Verification items for the finished model (mm, model axes). A direction names the side the tool comes from. Round coordinates to 2 decimals unless told otherwise and drop trailing zeros. Order: outer loops, then holes, each group sorted by start corner. A loop starts at its lowest first (then second) coordinate and runs counter-clockwise, first axis right, second up. Notation, with made-up numbers: M 42.25,44 L 67.25,44 A29 cw 67.25,64 Z; hole C 51,60 d1. An arc over 180 degrees is marked long. Return JSON: item names as keys, results as strings. Group by question number.
from build123d import *

# Parameters (mm, degrees)
BOSS_EXTRUDE1_DEPTH = 10
SKETCH1_3_R         = 7.5
BOSS_EXTRUDE2_DEPTH = 35
SKETCH3_W           = 111
SKETCH3_H           = 10
BOSS_EXTRUDE3_DEPTH = 300
SKETCH4_R           = 5
BOSS_EXTRUDE4_DEPTH = 15


with BuildPart() as part:
    # Sketch1 → Boss-Extrude1 (new body)
    with BuildSketch(Plane.XY):
        Polygon((30, 0), (30, 50), (-30, 50), (-30, 0), (-10.143306561, -30), (10.143306561, -30), align=None)
    boss_extrude1 = extrude(amount=BOSS_EXTRUDE1_DEPTH)

    # Sketch1_3 → Boss-Extrude2 (add)
    with BuildSketch(Plane.XY):
        Circle(SKETCH1_3_R)
    boss_extrude2 = extrude(amount=-BOSS_EXTRUDE2_DEPTH)

    # Sketch3 → Boss-Extrude3 (add)
    with BuildSketch(Plane.XY.offset(10)):
        with Locations((0, 55)):
            Rectangle(SKETCH3_W, SKETCH3_H)
    boss_extrude3 = extrude(amount=-BOSS_EXTRUDE3_DEPTH)

    # Mirror1: Boss-Extrude1, Boss-Extrude2, Boss-Extrude3 across plane
    add(boss_extrude1.mirror(Plane(origin=(0, 0, -290), x_dir=(1, 0, 0), z_dir=(0, 0, -1))))
    add(boss_extrude2.mirror(Plane(origin=(0, 0, -290), x_dir=(1, 0, 0), z_dir=(0, 0, -1))))
    add(boss_extrude3.mirror(Plane(origin=(0, 0, -290), x_dir=(1, 0, 0), z_dir=(0, 0, -1))))

    # Sketch4 → Boss-Extrude4 (add)
    with BuildSketch(Plane(origin=(0, 60, 0), x_dir=(1, 0, 0), z_dir=(0, 1, 0))):
        with Locations(Location((-45.5, -2.5, 0), (0, 0, 180))):
            Circle(SKETCH4_R)
        with Locations(Location((45.5, -2.5, 0), (0, 0, 180))):
            Circle(SKETCH4_R)
        with Locations(Location((-45.5, 552.5, 0), (0, 0, 180))):
            Circle(SKETCH4_R)
        with Locations(Location((45.5, 552.5, 0), (0, 0, 180))):
            Circle(SKETCH4_R)
    extrude(amount=BOSS_EXTRUDE4_DEPTH)


solid = part.part
1. Access from +Z, -Z, +X, -X, +Y, -Y to the whole of each face (thin tool, end or side, straight path). Record for faces 4 (the face through (30, 25, 5)), 5 (the face through (46.151, 67.395, -547.543)), 6 (the face through (-30, 25, 5)), 7 (the face through (-45, 75, -552)), 8 (the face through (55.5, 55, -294)).
2. Go/stop test with flat-tipped pins: pin 1 (3 mm diameter, centred on y = 18, z = 5.5, fed in from -X); pin 2 (6 mm diameter, centred on x = 8, z = -401, fed in from -Y); pin 3 (5 mm diameter, centred on y = 18, z = 5.5, fed in from +X). Record where each tip stops, or that it passes through.
3. Cross-section at A-A (z = -552.5). Enter the section's corners in (x, y), plus the area to 3 significant figures.
4. Draft check along Z on faces 1 (the face through (-1, 26, 10)), 2 (the face through (-30, 25, -585)), 3 (the face through (-7.493, 0.33, -562.745)). Enter one of: +Z half, -Z half, draft (parallel to the pull), parting line (faces both ways), or undercut.
5. Cross-section at D-D (y = 67). Enter the section's corners in (x, z).
6. Thickness scan on line 1 along Z through (x, y) = (13, -2.5); line 2 along Z through (x, y) = (-1, -4); line 3 along Y through (x, z) = (40.5, -496). Record the ranges inside material, lowest first. Write a range as from..to.
7. Cross-section at C-C (x = 45.5). Enter the section's corners in (y, z), plus the area to 3 significant figures.
8. Cross-section at B-B (y = 16). Enter the section's corners in (x, z).
Computed:
{
 "1": {"face 4": "+Z, -Z, +X, -Y", "face 5": "+Y", "face 6": "+Z, -Z, -X, -Y", "face 7": "+Z, -Z, +X, -X, +Y", "face 8": "+Z, -Z, +X, +Y, -Y"},
 "2": {"pin 1": "stops at x = -30", "pin 2": "stops at y = 50", "pin 3": "stops at x = 30"},
 "3": {"outline": "M -55.5,50 L 55.5,50 L 55.5,60 L 50.5,60 L 50.5,75 L 40.5,75 L 40.5,60 L -40.5,60 L -40.5,75 L -50.5,75 L -50.5,60 L -55.5,60 Z; C 0,0 d15", "area": "1,590 mm²"},
 "4": {"face 1": "+Z half", "face 2": "draft", "face 3": "undercut"},
 "5": {"outline": "C -45.5,-552.5 d10; C -45.5,2.5 d10; C 45.5,-552.5 d10; C 45.5,2.5 d10"},
 "6": {"line 1": "z = -590..-580, 0..10", "line 2": "z = -590..-545, -35..10", "line 3": "y = 50..60"},
 "7": {"outline": "M 50,-590 L 60,-590 L 60,-557.5 L 75,-557.5 L 75,-547.5 L 60,-547.5 L 60,-2.5 L 75,-2.5 L 75,7.5 L 60,7.5 L 60,10 L 50,10 Z", "area": "6,300 mm²"},
 "8": {"outline": "M -30,-590 L 30,-590 L 30,-580 L -30,-580 Z; M -30,0 L 30,0 L 30,10 L -30,10 Z"}
}
